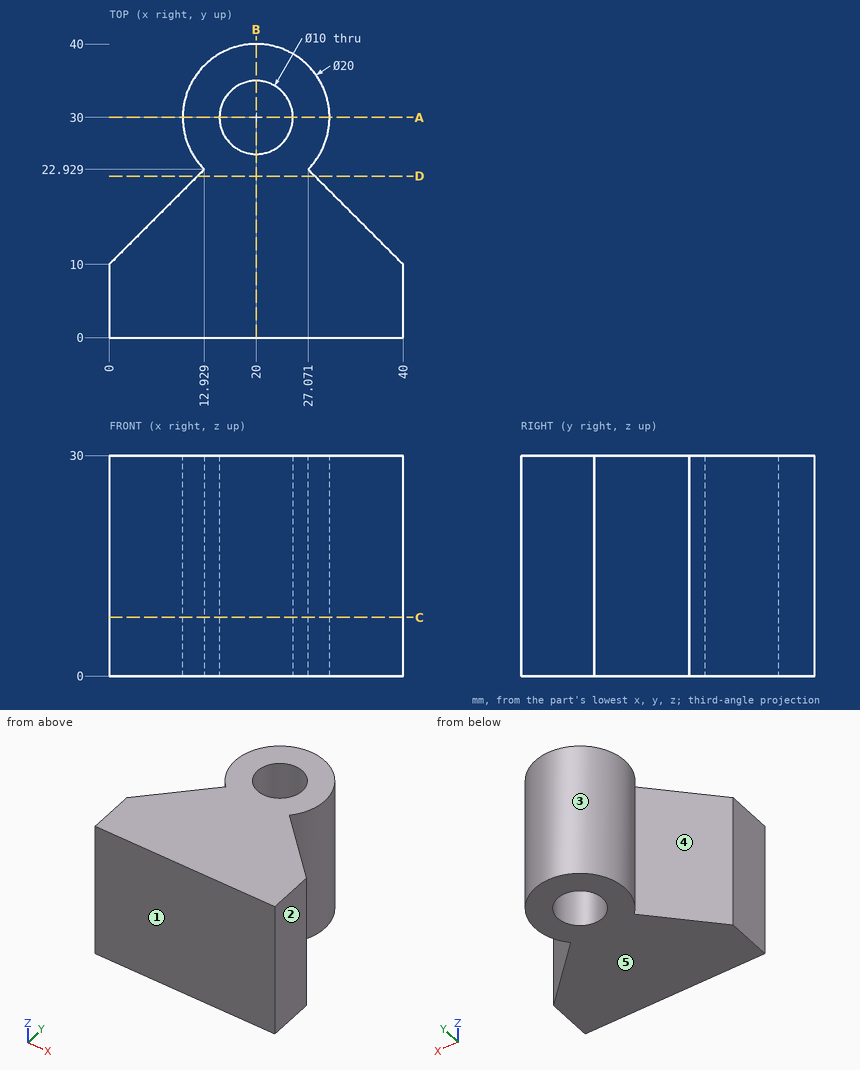
Geometry check sheet. Reference: drawing and pictorial views, mm from the part's lowest x, y, z. A direction names the side the tool comes from. Give positions to 0.01 mm unless a question says otherwise; leave off trailing zeros. Order: outer loops, then holes, each group sorted by start corner. A loop starts at its lowest first (then second) coordinate and runs counter-clockwise, first axis right, second up. Notation, with made-up numbers: M 14.25,20.25 L 57.25,20.25 A12 ccw 57.25,24.25 Z; hole C 17,13 d9. An arc over 180 degrees is marked long. Answer in a Markdown table with one row per item.
1) Cross-section at D-D, the plane y = 22. Enter the section's corners in (x, z).
Filled sheet:
| item | result |
|---|---|
| outline | M 12,0 L 28,0 L 28,30 L 12,30 Z |
2) Release check for a two-part mould opening along Y. For the marked faces 1, 2 and 3 record: +Y half, -Y half, draft (parallel to the pull), parting line (faces both ways), or undercut.
Filled sheet:
| item | result |
|---|---|
| face 1 | -Y half |
| face 2 | draft |
| face 3 | undercut |
3) Cross-section at A-A, the plane y = 30. Enter the section's corners in (x, z), plus the area to 3 significant figures.
Filled sheet:
| item | result |
|---|---|
| outline | M 10,0 L 15,0 L 15,30 L 10,30 Z; M 25,0 L 30,0 L 30,30 L 25,30 Z |
| area | 300 mm2 |
4) Cross-section at C-C, the plane z = 8. Enter the section's corners in (x, y), plus the area to 3 significant figures.
Filled sheet:
| item | result |
|---|---|
| outline | M 0,0 L 40,0 L 40,10 L 27.07,22.93 A10 ccw long 12.93,22.93 L 0,10 Z; hole C 20,30 d10 |
| area | 957 mm2 |
5) Cross-section at B-B, the plane x = 20. Enter the section's corners in (y, z), plus the area to 3 significant figures.
Filled sheet:
| item | result |
|---|---|
| outline | M 0,0 L 25,0 L 25,30 L 0,30 Z; M 35,0 L 40,0 L 40,30 L 35,30 Z |
| area | 900 mm2 |
6) Thickness scan on L1, parallel to Y at x = 12, z = 18.75; L2, parallel to X at y = 30.5, z = 20.25 (1 decimal); L3, parallel to X at y = 28.5, z = 6.5. Record the ranges inside material, lowest first. Write a range as [from, to].
Filled sheet:
| item | result |
|---|---|
| L1 | y = [0, 22], [24, 36] |
| L2 | x = [10, 15], [25, 30] |
| L3 | x = [10.11, 15.23], [24.77, 29.89] |
7) Gauge pin test, flat ends, axial feed: P1, Ø1, axis at y = 14, z = 26.5, coming from the -X side; P2, Ø1.5, axis at y = 11, z = 17, coming from the +X side; P3, Ø6, axis at y = 30, z = 8, coming from the +X side. Record the tip position at first contact, or that the pin passes through.
Filled sheet:
| item | result |
|---|---|
| P1 | stops at x = 3.5 |
| P2 | stops at x = 39.75 |
| P3 | stops at x = 30 |
8) Access from +Z, -Z, +X, -X, +Y, -Y to the whole of each face (thin tool, end or side, straight path). Record for the marked faces 4 and 5.
Filled sheet:
| item | result |
|---|---|
| face 4 | +Z, -Z, -X |
| face 5 | -Z, +X, -X, +Y, -Y |
